```python
from build123d import *

# Parameters (mm, degrees)
SKETCH1_R           = 3.2385
BOSS_EXTRUDE1_DEPTH = 8.255
BOSS_EXTRUDE2_DEPTH = 1.4605
SKETCH3_R           = 1.6256
CUT_EXTRUDE1_DEPTH  = 21.180615699
CUT_EXTRUDE2_DEPTH  = 42.211451079
SKETCH6_W           = 16.51
SKETCH6_H           = 6.731
BOSS_EXTRUDE3_DEPTH = 1.905
SKETCH5_R           = 2.2225
CUT_EXTRUDE3_DEPTH  = 6.35
FILLET1_R           = 1.27
FILLET2_R           = 2.54


with BuildPart() as part:
    # Sketch1 → Boss-Extrude1 (new, symmetric)
    with BuildSketch(Plane(origin=(0, 0, 0), x_dir=(0, 0, -1), z_dir=(1, 0, 0))):
        with BuildLine():
            Line((12.7, 19.05), (-12.7, 19.05))
            Line((-12.7, 19.05), (-12.7, 22.225))
            Line((-12.7, 22.225), (-6.35, 22.225))
            Line((-6.35, 22.225), (-6.35, 29.21))
            ThreePointArc((-6.35, 29.21), (0, 35.56), (6.35, 29.21))
            Line((6.35, 29.21), (6.35, 22.225))
            Line((6.35, 22.225), (12.7, 22.225))
            Line((12.7, 22.225), (12.7, 19.05))
        make_face()
        with Locations((0, 29.21)):
            Circle(SKETCH1_R, mode=Mode.SUBTRACT)
    extrude(amount=BOSS_EXTRUDE1_DEPTH, both=True)

    # Sketch2 → Boss-Extrude2 (add, symmetric)
    with BuildSketch(Plane(origin=(0, 0, 0), x_dir=(0, 0, -1), z_dir=(1, 0, 0))):
        Polygon((-5.499261314, 32.385), (-12.7, 22.225), (-5.499261314, 22.225), align=None)
        Polygon((5.499261314, 22.225), (5.499261314, 32.385), (12.7, 22.225), align=None)
    extrude(amount=BOSS_EXTRUDE2_DEPTH, both=True)

    # Sketch3 → Cut-Extrude1 (cut, through all)
    with BuildSketch(Plane(origin=(0, 22.225, 0), x_dir=(1, 0, 0), z_dir=(0, 1, 0))):
        with Locations(Location((-5.08, 9.525, 0), (0, 0, 270))):
            Circle(SKETCH3_R)
        with Locations(Location((5.08, 9.525, 0), (0, 0, 90))):
            Circle(SKETCH3_R)
        with Locations(Location((5.08, -9.525, 0), (0, 0, 270))):
            Circle(SKETCH3_R)
        with Locations(Location((-5.08, -9.525, 0), (0, 0, 90))):
            Circle(SKETCH3_R)
    extrude(amount=-CUT_EXTRUDE1_DEPTH, mode=Mode.SUBTRACT)

    # Sketch4 → Cut-Extrude2 (cut, through all)
    with BuildSketch(Plane(origin=(8.255, 0, 0), x_dir=(0, 0, -1), z_dir=(1, 0, 0))):
        with BuildLine():
            Line((3.3655, 34.594785024), (-3.3655, 34.594785024))
            ThreePointArc((-3.3655, 34.594785024), (0, 35.56), (3.3655, 34.594785024))
        make_face()
    extrude(amount=-CUT_EXTRUDE2_DEPTH, mode=Mode.SUBTRACT)

    # Sketch6 → Boss-Extrude3 (add)
    with BuildSketch(Plane(origin=(0, 34.594785024, 0), x_dir=(1, 0, 0), z_dir=(0, 1, 0))):
        Rectangle(SKETCH6_W, SKETCH6_H)
    extrude(amount=BOSS_EXTRUDE3_DEPTH)

    # Sketch5 → Cut-Extrude3 (cut)
    with BuildSketch(Plane(origin=(0, 36.499785024, 0), x_dir=(1, 0, 0), z_dir=(0, 1, 0))):
        with Locations(Location((-4.445, 0, 0), (0, 0, 270))):
            Circle(SKETCH5_R)
        with Locations(Location((4.445, 0, 0), (0, 0, 270))):
            Circle(SKETCH5_R)
    extrude(amount=-CUT_EXTRUDE3_DEPTH, mode=Mode.SUBTRACT)

    # Fillet1
    fillet1_edges = [part.edges().sort_by_distance(p)[0] for p in [
        (-8.255, 20.6375, -12.7),
        (-8.255, 20.6375, 12.7),
        (8.255, 20.6375, -12.7),
        (1.4605, 25.7175, 6.35),
        (1.4605, 30.853500936, 6.133628997),
        (-1.4605, 25.7175, 6.35),
        (-1.4605, 30.853500936, 6.133628997),
        (-1.4605, 25.7175, -6.35),
        (1.4605, 25.7175, -6.35),
        (8.255, 20.6375, 12.7),
        (1.4605, 30.853500936, -6.133628997),
        (-1.4605, 30.853500936, -6.133628997),
    ]]
    fillet(fillet1_edges, radius=FILLET1_R)

    # Fillet2
    fillet2_edges = [part.edges().sort_by_distance(p)[0] for p in [
        (0, 34.594785024, 3.3655),
        (0, 34.594785024, -3.3655),
    ]]
    fillet(fillet2_edges, radius=FILLET2_R)


solid = part.part
```
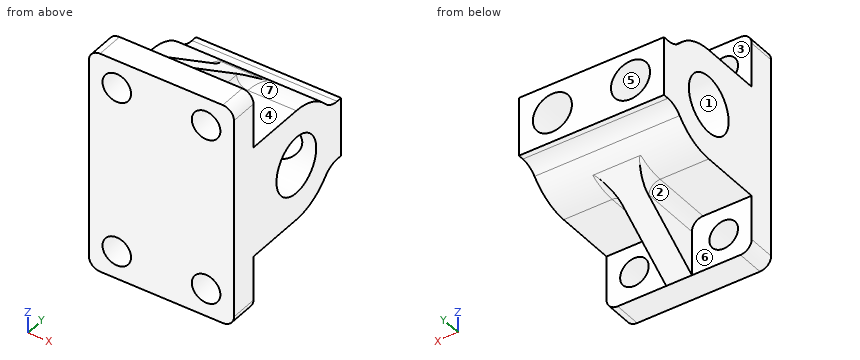
Work out the finished part from the listing and answer in its coordinate system (mm). Face numbers are marked on the shaded views. A direction names the side the tool comes from. Coordinates: 2 decimals unless noted, no trailing zeros. Loops run counter-clockwise (first coordinate to the right, second up) from the corner with the lowest first, then second, coordinate; pieces in that order, holes last. Notation, with made-up numbers: (-2.5, -21) - (18.5, -21) arc R20 ccw to (18.5, -7) - close; hole circle Ø9 at (83.5, 0). An arc over 180 degrees is marked (long way). Use a Markdown table: item, result.
Item 1: For the marked faces 4, 5, 6 and 7, determine the directions among +Z, -Z, +X, -X, +Y, -Y from which every point of the face is accessible in a straight line to the end or side of a thin tool.
Evaluation:
| item | result |
|---|---|
| face 4 | +Z, +X, +Y |
| face 5 | +Y |
| face 6 | -Z, -X, +Y |
| face 7 | +Z, +Y |
Item 2: Given pin 1 Ø3 at (x, z) = (3.5, 10.5) entering from +Y (3 decimals); pin 2 Ø6 at (x, y) = (-6.5, 27.5) entering from -Z; pin 3 Ø2.5 at (y, z) = (25, -9) entering from +X, each flat-ended and moving along its own axis, determine where each tip first touches the part or whether it passes through.
Evaluation:
| item | result |
|---|---|
| pin 1 | stops at y = 22.225 |
| pin 2 | stops at z = -6.35 |
| pin 3 | stops at x = 1.46 |
Item 3: Find section B-B, the plane y = 21.5. Determine the outline of the cut face in (x, z) (3 decimals).
Evaluation:
| item | result |
|---|---|
| outline | (-8.255, -11.43) arc R1.27 ccw to (-6.985, -12.7) - (6.985, -12.7) arc R1.27 ccw to (8.255, -11.43) - (8.255, 11.43) arc R1.27 ccw to (6.985, 12.7) - (-6.985, 12.7) arc R1.27 ccw to (-8.255, 11.43) - close; hole circle Ø3.251 at (-5.08, -9.525); hole circle Ø3.251 at (-5.08, 9.525); hole circle Ø3.251 at (5.08, -9.525); hole circle Ø3.251 at (5.08, 9.525) |
Item 4: The mould has two halves that part along Z. Classify the marked faces 1, 2 and 3: +Z half, -Z half, draft (parallel to the pull), parting line (faces both ways), or undercut.
Evaluation:
| item | result |
|---|---|
| face 1 | undercut |
| face 2 | -Z half |
| face 3 | draft |
Item 5: Consider probe 1 along X at (y, z) = (22, 8.25) (3 decimals); probe 2 along Z at (x, y) = (-4, 20.25); probe 3 along Y at (x, z) = (-0.25, 0). Determine where each line is inside the solid, lowest interval first. Write a range as from..to.
Evaluation:
| item | result |
|---|---|
| probe 1 | x = -8.255..-6.088, -4.072..4.072, 6.088..8.255 |
| probe 2 | z = -12.7..-10.74, -8.31..8.31, 10.74..12.7 |
| probe 3 | y = 19.05..25.97, 32.45..36.5 |
Item 6: Find section A-A, the plane z = 0. State how many separate pieces and enclosed holes the cut face has, and give its area (3 significant figures).
Evaluation:
| item | result |
|---|---|
| separate pieces | 4 |
| enclosed holes | 0 |
| area | 145 mm2 |
